Geometry: final body of the model. Coordinates: model frame, mm. Coordinates: 2 decimals unless noted, no trailing zeros. Order: outer loops, then holes, each group sorted by start corner. A loop starts at its lowest first (then second) coordinate and runs counter-clockwise, first axis right, second up. Notation, with made-up numbers: (-29, -20.75) -> (26, -20.75) arc R11 ccw to (26, -12.75) -> close; hole circle Ø2 at (23, 11). An arc over 180 degrees is marked (long way). Use CSV: the item, a comma, the result in double quotes. Start each with the question number.
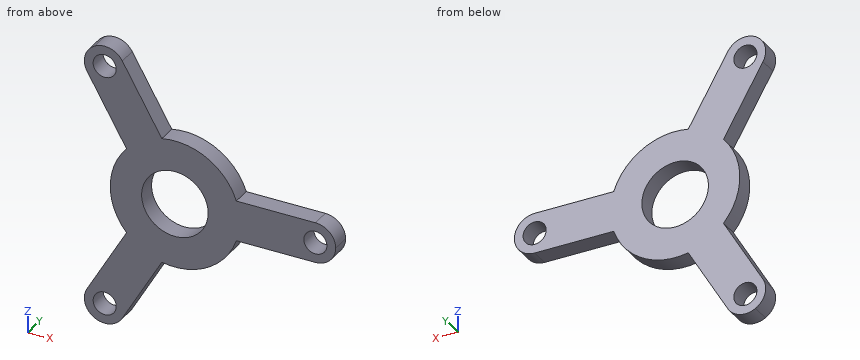
from build123d import *

# Parameters (mm, degrees)
SKETCH1_R           = 17.5
SKETCH1_R_2         = 9
BOSS_EXTRUDE1_DEPTH = 5
BOSS_EXTRUDE3_DEPTH = 5
CUT_EXTRUDE1_START  = -6
SKETCH4_R           = 3.125
CUT_EXTRUDE1_DEPTH  = 7
CIRPATTERN1_COUNT   = 3


with BuildPart() as part:
    # Sketch1 → Boss-Extrude1 (new body)
    with BuildSketch(Plane(origin=(0, 0, 0), x_dir=(1, 0, 0), z_dir=(0, 1, 0))):
        Circle(SKETCH1_R)
        Circle(SKETCH1_R_2, mode=Mode.SUBTRACT)
    extrude(amount=BOSS_EXTRUDE1_DEPTH)

    # Sketch3 → Boss-Extrude3 (add)
    with BuildSketch(Plane(origin=(0, 0, 0), x_dir=(1, 0, 0), z_dir=(0, 1, 0))):
        with BuildLine():
            Line((38, 5.5), (10.009906254, 5.5))
            Line((10.009906254, 5.5), (10.009906254, -5.5))
            Line((10.009906254, -5.5), (38, -5.5))
            ThreePointArc((38, -5.5), (32.5, 0), (38, 5.5))
        make_face()
        with BuildLine():
            ThreePointArc((43.5, 0), (41.889087297, 3.889087297), (38, 5.5))
            Line((38, 5.5), (38, -5.5))
            ThreePointArc((38, -5.5), (41.889087297, -3.889087297), (43.5, 0))
        make_face()
        with BuildLine():
            Line((38, -5.5), (38, 5.5))
            ThreePointArc((38, 5.5), (32.5, 0), (38, -5.5))
        make_face()
    boss_extrude3 = extrude(amount=BOSS_EXTRUDE3_DEPTH)

    # Sketch4 → Cut-Extrude1 (cut)
    with BuildSketch(Plane(origin=(0, 5, 0), x_dir=(1, 0, 0), z_dir=(0, 1, 0)).offset(CUT_EXTRUDE1_START)):
        with Locations((38, 0)):
            Circle(SKETCH4_R)
    cut_extrude1 = extrude(amount=CUT_EXTRUDE1_DEPTH, mode=Mode.SUBTRACT)

    # CirPattern1: Boss-Extrude3, Cut-Extrude1 ×3 about axis
    cirpattern1_axis = Axis((0, 0, 0), (0, 1, 0))
    for i in range(1, CIRPATTERN1_COUNT):
        add(boss_extrude3.rotate(cirpattern1_axis, i * 360 / CIRPATTERN1_COUNT))
        add(cut_extrude1.rotate(cirpattern1_axis, i * 360 / CIRPATTERN1_COUNT), mode=Mode.SUBTRACT)


solid = part.part
(1) Line query: line 1 (Z direction, x = 38, y = 1) (3 decimals); line 2 (Z direction, x = 0, y = 3.6); line 3 (Z direction, x = -19, y = 2.95). Output: solid intervals per line, ascending. Write a range as from..to.
(2) Section B-B (x = -19). Return loops of the section in (y, z).
(3) First-contact query: pin 1 (1 mm diameter, centred on x = 18, y = 2.5, fed in from +Z); pin 2 (1.5 mm diameter, centred on y = 3.5, z = -12, fed in from -X); pin 3 (1 mm diameter, centred on x = 2.5, y = 4, fed in from -Z). Flat tips, straight axial feed; report the tip coordinate or a pass-through.
(4) Section D-D (z = 21). Return loops of the section in (x, y), then the cut area to 3 significant figures.
(5) Section A-A (x = 0). Return loops of the section in (y, z), then the cut area to 3 significant figures.
(6) Section C-C (y = 2.45). State how many separate pieces and enclosed holes the cut face has, then the cut area to 3 significant figures.
Check sheet entries:
1,line 1,"z = -5.5..-3.125, 3.125..5.5"
1,line 2,"z = -17.5..-9, 9..17.5"
1,line 3,"z = -38.41..-36.03, -29.78..-21.91, 21.91..29.78, 36.03..38.41"
2,outline,"(0, -38.41) -> (5, -38.41) -> (5, -36.03) -> (0, -36.03) -> close; (0, -29.78) -> (5, -29.78) -> (5, -21.91) -> (0, -21.91) -> close; (0, 21.91) -> (5, 21.91) -> (5, 29.78) -> (0, 29.78) -> close; (0, 36.03) -> (5, 36.03) -> (5, 38.41) -> (0, 38.41) -> close"
3,pin 1,"stops at z = 5.5"
3,pin 2,"stops at x = -13.71"
3,pin 3,"stops at z = -17.39"
4,outline,"(-18.48, 0) -> (-5.77, 0) -> (-5.77, 5) -> (-18.48, 5) -> close"
4,area,"63.5 mm^2"
5,outline,"(0, -17.5) -> (5, -17.5) -> (5, -9) -> (0, -9) -> close; (0, 9) -> (5, 9) -> (5, 17.5) -> (0, 17.5) -> close"
5,area,"85.0 mm^2"
6,separate pieces,"1"
6,enclosed holes,"4"
6,area,"1,440 mm^2"
